from build123d import *

# Parameters (mm, degrees)
SKETCH_1_W      = 960
SKETCH_1_H      = 550
EXTRUDE_1_DEPTH = 12
SKETCH_2_W      = 640
SKETCH_2_H      = 162.5
EXTRUDE_2_DEPTH = 12
SKETCH_3_W      = 640
SKETCH_3_H      = 162.5
EXTRUDE_3_DEPTH = 12
SKETCH_4_W      = 12.5
SKETCH_4_H      = 526
EXTRUDE_4_DEPTH = 162.5


with BuildPart() as part:
    # 草图1 → 凸台-拉伸1 (new body)
    with BuildSketch(Plane.XY):
        with Locations((480, 275)):
            Rectangle(SKETCH_1_W, SKETCH_1_H)
    extrude(amount=EXTRUDE_1_DEPTH)

    # 草图2 → 凸台-拉伸2 (add)
    with BuildSketch(Plane(origin=(0, 550, 0), x_dir=(1, 0, 0), z_dir=(0, 1, 0))):
        with Locations((480, -6)):
            Rectangle(SKETCH_2_W, SKETCH_2_H)
    extrude(amount=-EXTRUDE_2_DEPTH)

    # 草图3 → 凸台-拉伸3 (add)
    with BuildSketch(Plane.XZ):
        with Locations((480, 6)):
            Rectangle(SKETCH_3_W, SKETCH_3_H)
    extrude(amount=-EXTRUDE_3_DEPTH)

    # 草图4 → 凸台-拉伸4 (add)
    with BuildSketch(Plane(origin=(0, 0, -75.25), x_dir=(-1, 0, 0), z_dir=(0, 0, -1))):
        with Locations((-600, 275)):
            Rectangle(SKETCH_4_W, SKETCH_4_H)
        with Locations((-360, 275)):
            Rectangle(SKETCH_4_W, SKETCH_4_H)
    extrude(amount=-EXTRUDE_4_DEPTH)


solid = part.part
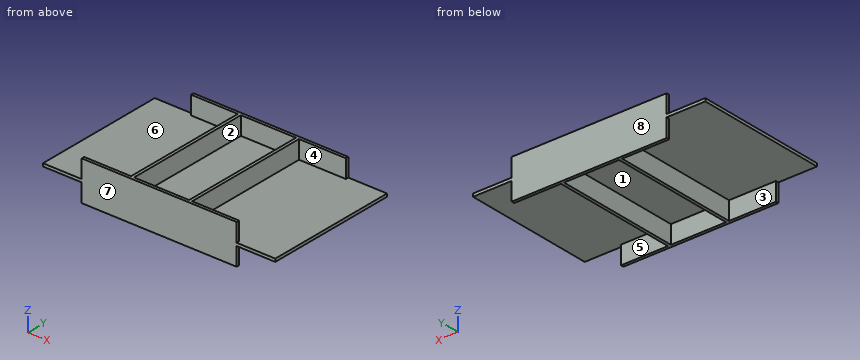
Could you check a few things on this model? Use its own coordinates, in mm. Face numbers are marked on the shaded views. A direction names the side the tool comes from. Give positions to 0.01 mm unless a question says otherwise; leave off trailing zeros. Order: outer loops, then holes, each group sorted by start corner. A loop starts at its lowest first (then second) coordinate and runs counter-clockwise, first axis right, second up. Notation, with made-up numbers: (-37, 67.25) -> (14, 67.25) arc R31 ccw to (14, 93.25) -> close; hole circle Ø5 at (22.25, -35.5). An arc over 180 degrees is marked (long way). Answer in a Markdown table with one row per item. Add a question column.
Item 1: Imagine slicing it at B-B (y = 91.5). List the corners of the cut face in (x, z) for me.
Item 2: I'm going to push flat-ended pins straight in: P1, Ø3.5, axis at y = 546.5, z = -41, coming from the +X side; P2, Ø2, axis at x = 493.5, y = 203, coming from the +Z side; P3, Ø5, axis at y = 322.5, z = 52.5, coming from the -X side. Where does each tip first touch, or does it pass through?
Item 3: Imagine slicing it at C-C (x = 509.5). List the corners of the cut face in (y, z) for me, and give its area (3 significant figures).
Item 4: Imagine slicing it at A-A (z = 45). List the corners of the cut face in (x, y) for me.
Item 5: We'd pull the mould along Y, two halves only. Please class the marked faces 6, 7 and 8: pulls with the +Y half, pulls with the -Y half, needs draft (parallel to the pull), parting line crosses it, or undercut.
Item 6: Please list where these lines run through material, in increasing order: probe 1 along Y at (x, z) = (379.5, 74); probe 2 along X at (y, z) = (456, -7.5); probe 3 along Z at (x, y) = (532, 139.5).
Item 7: Imagine slicing it at D-D (x = 810). List the corners of the cut face in (y, z) for me.
Item 8: For the marked faces 1, 2, 3, 4 and 5, which set-ups out of +Z, -Z, +X, -X, +Y, -Y let a thin tool reach every point of the face, with its end or its side?
Result:
| question | item | result |
|---|---|---|
| 1 | outline | (0, 0) -> (353.75, 0) -> (353.75, -75.25) -> (366.25, -75.25) -> (366.25, 0) -> (593.75, 0) -> (593.75, -75.25) -> (606.25, -75.25) -> (606.25, 0) -> (960, 0) -> (960, 12) -> (606.25, 12) -> (606.25, 87.25) -> (593.75, 87.25) -> (593.75, 12) -> (366.25, 12) -> (366.25, 87.25) -> (353.75, 87.25) -> (353.75, 12) -> (0, 12) -> close |
| 2 | P1 | x = 800 |
| 2 | P2 | z = 12 |
| 2 | P3 | x = 353.75 |
| 3 | outline | (0, -75.25) -> (12, -75.25) -> (12, 0) -> (538, 0) -> (538, -75.25) -> (550, -75.25) -> (550, 87.25) -> (538, 87.25) -> (538, 12) -> (12, 12) -> (12, 87.25) -> (0, 87.25) -> close |
| 3 | area | 10,200 mm2 |
| 4 | outline | (160, 0) -> (800, 0) -> (800, 12) -> (606.25, 12) -> (606.25, 538) -> (800, 538) -> (800, 550) -> (160, 550) -> (160, 538) -> (353.75, 538) -> (353.75, 12) -> (160, 12) -> close; hole (366.25, 12) -> (593.75, 12) -> (593.75, 538) -> (366.25, 538) -> close |
| 5 | face 6 | undercut |
| 5 | face 7 | pulls with the -Y half |
| 5 | face 8 | pulls with the +Y half |
| 6 | probe 1 | 0 to 12, 538 to 550 |
| 6 | probe 2 | 353.75 to 366.25, 593.75 to 606.25 |
| 6 | probe 3 | 0 to 12 |
| 7 | outline | (0, 0) -> (550, 0) -> (550, 12) -> (0, 12) -> close |
| 8 | face 1 | -Z |
| 8 | face 2 | +Z |
| 8 | face 3 | -Z, -X |
| 8 | face 4 | +Z, +X |
| 8 | face 5 | -Z, +X |
